```python
from build123d import *

# Parameters (mm, degrees)
ESBO_O1_R                    = 100
ESBO_O1_R_2                  = 27.5
RESSALTO_EXTRUS_O1_DEPTH     = 65
CORTE_EXTRUS_O1_START        = -5
ESBO_O2_R                    = 100
ESBO_O2_R_2                  = 42.5
CORTE_EXTRUS_O1_DEPTH        = 55
CORTE_EXTRUS_O2_DEPTH        = 157.3
FILETE1_R                    = 10
PADR_OCIRCULAR1_COUNT        = 6
FILETE1_OF_PADR_OCIRCULAR1_R = 10
ESBO_O4_R                    = 4
CORTE_EXTRUS_O3_DEPTH        = 157.3
PADR_OCIRCULAR2_COUNT        = 22


with BuildPart() as part:
    # Esboço1 → Ressalto-extrusão1 (new body)
    with BuildSketch(Plane.XY):
        Circle(ESBO_O1_R)
        Circle(ESBO_O1_R_2, mode=Mode.SUBTRACT)
    extrude(amount=RESSALTO_EXTRUS_O1_DEPTH)

    # Esboço2 → Corte-extrusão1 (cut)
    with BuildSketch(Plane.XY.offset(65).offset(CORTE_EXTRUS_O1_START)):
        Circle(ESBO_O2_R)
        Circle(ESBO_O2_R_2, mode=Mode.SUBTRACT)
    extrude(amount=-CORTE_EXTRUS_O1_DEPTH, mode=Mode.SUBTRACT)

    # Esboço3 → Corte-extrusão2 (cut)
    with BuildSketch(Plane.XY.offset(65)):
        with BuildLine():
            ThreePointArc((0, 87.5), (-33.484800332, 80.839459095), (-61.871843354, 61.871843354))
            Line((-61.871843354, 61.871843354), (-32.082845763, 44.673157576))
            ThreePointArc((-32.082845763, 44.673157576), (-21.04758878, 50.813374288), (-8.90269486, 54.274690457))
            Line((-8.90269486, 54.274690457), (0, 87.5))
        make_face()
    corte_extrus_o2 = extrude(amount=-CORTE_EXTRUS_O2_DEPTH, mode=Mode.SUBTRACT)

    # Filete1
    filete1_edges = [part.edges().sort_by_distance(p)[0] for p in [
        (0, 87.5, 2.5),
        (0, 87.5, 62.5),
        (-8.90269486, 54.274690457, 2.5),
        (-8.90269486, 54.274690457, 62.5),
        (-32.082845763, 44.673157576, 2.5),
        (-32.082845763, 44.673157576, 62.5),
        (-61.871843354, 61.871843354, 2.5),
        (-61.871843354, 61.871843354, 62.5),
    ]]
    fillet(filete1_edges, radius=FILETE1_R)

    # PadrãoCircular1: Corte-extrusão2 ×6 about axis
    padr_ocircular1_axis = Axis((0, 0, 0), (0, 0, 1))
    for i in range(1, PADR_OCIRCULAR1_COUNT):
        add(corte_extrus_o2.rotate(padr_ocircular1_axis, i * 360 / PADR_OCIRCULAR1_COUNT), mode=Mode.SUBTRACT)

    # Filete1 of PadrãoCircular1
    filete1_of_padr_ocircular1_edges = [part.edges().sort_by_distance(p)[0] for p in [
        (-75.777222831, 43.75, 2.5),
        (-75.777222831, 43.75, 62.5),
        (-51.454608149, 19.427385317, 2.5),
        (-51.454608149, 19.427385317, 62.5),
        (-54.729512209, -5.447980668, 2.5),
        (-54.729512209, -5.447980668, 62.5),
        (-84.5185098, -22.646666446, 2.5),
        (-84.5185098, -22.646666446, 62.5),
        (-75.777222831, -43.75, 2.5),
        (-75.777222831, -43.75, 62.5),
        (-42.551913288, -34.84730514, 2.5),
        (-42.551913288, -34.84730514, 62.5),
        (-22.646666446, -50.121138244, 2.5),
        (-22.646666446, -50.121138244, 62.5),
        (-22.646666446, -84.5185098, 2.5),
        (-22.646666446, -84.5185098, 62.5),
        (0, -87.5, 2.5),
        (0, -87.5, 62.5),
        (8.90269486, -54.274690457, 2.5),
        (8.90269486, -54.274690457, 62.5),
        (32.082845763, -44.673157576, 2.5),
        (32.082845763, -44.673157576, 62.5),
        (61.871843354, -61.871843354, 2.5),
        (61.871843354, -61.871843354, 62.5),
        (75.777222831, -43.75, 2.5),
        (75.777222831, -43.75, 62.5),
        (51.454608149, -19.427385317, 2.5),
        (51.454608149, -19.427385317, 62.5),
        (54.729512209, 5.447980668, 2.5),
        (54.729512209, 5.447980668, 62.5),
        (84.5185098, 22.646666446, 2.5),
        (84.5185098, 22.646666446, 62.5),
        (75.777222831, 43.75, 2.5),
        (75.777222831, 43.75, 62.5),
        (42.551913288, 34.84730514, 2.5),
        (42.551913288, 34.84730514, 62.5),
        (22.646666446, 50.121138244, 2.5),
        (22.646666446, 50.121138244, 62.5),
        (22.646666446, 84.5185098, 2.5),
        (22.646666446, 84.5185098, 62.5),
    ]]
    fillet(filete1_of_padr_ocircular1_edges, radius=FILETE1_OF_PADR_OCIRCULAR1_R)

    # Esboço4 → Corte-extrusão3 (cut)
    with BuildSketch(Plane.XY.offset(65)):
        with Locations((0, 35)):
            Circle(ESBO_O4_R)
    corte_extrus_o3 = extrude(amount=-CORTE_EXTRUS_O3_DEPTH, mode=Mode.SUBTRACT)

    # PadrãoCircular2: Corte-extrusão3 ×22 about axis
    padr_ocircular2_axis = Axis((0, 0, 0), (0, 0, 1))
    for i in range(1, PADR_OCIRCULAR2_COUNT):
        add(corte_extrus_o3.rotate(padr_ocircular2_axis, i * 360 / PADR_OCIRCULAR2_COUNT), mode=Mode.SUBTRACT)


solid = part.part
```
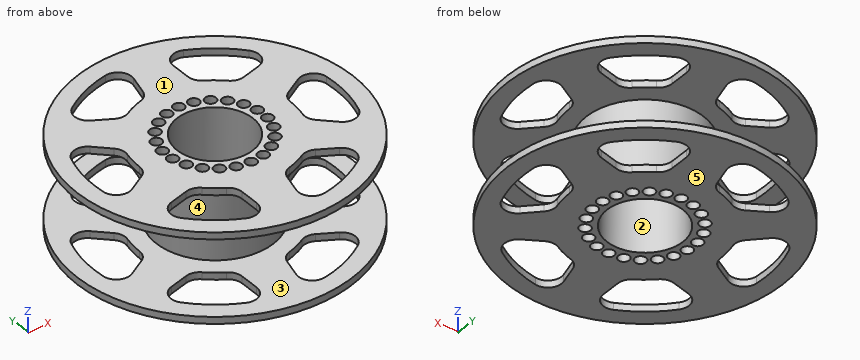
Here's how the part is built. I have some questions about the finished solid (model axes, mm). Face numbers are marked on the shaded views. A direction names the side the tool comes from. Round coordinates to 2 decimals unless told otherwise and drop trailing zeros. Order: outer loops, then holes, each group sorted by start corner. A loop starts at its lowest first (then second) coordinate and runs counter-clockwise, first axis right, second up. Notation, with made-up numbers: M 6,-15 L 61,-15 A23 cw 61,19 Z; hole C -6.75,8.5 d11. An arc over 180 degrees is marked long. Answer in a Markdown table with one row per item.
Item 1: If I drill on L1, parallel to Z at x = -27.5, y = 42.5; L2, parallel to Y at x = 35, z = 38.5; L3, parallel to Y at x = 21.5, z = 56.5, over which ranges is the centre line in solid material (lowest first)? Write a range as from..to.
A:
| item | result |
|---|---|
| L1 | z = 0..5, 60..65 |
| L2 | y = -24.11..-16.99, -12.09..-8.97, -1..1, 8.97..12.09, 16.99..24.11 |
| L3 | y = -36.66..-32.5, -26.39..-17.15, 17.15..26.39, 32.5..36.66 |
Item 2: Imagine slicing it at B-B, the plane y = 77. Write out the boundary of the cut face in (x, z).
A:
| item | result |
|---|---|
| outline | M -63.8,0 L -41.56,0 L -41.56,5 L -63.8,5 Z; M -63.8,60 L -41.56,60 L -41.56,65 L -63.8,65 Z; M -3.36,0 L 25.23,0 L 25.23,5 L -3.36,5 Z; M -3.36,60 L 25.23,60 L 25.23,65 L -3.36,65 Z; M 41.56,0 L 63.8,0 L 63.8,5 L 41.56,5 Z; M 41.56,60 L 63.8,60 L 63.8,65 L 41.56,65 Z |
Item 3: For the marked faces 4 and 5, which set-ups out of +Z, -Z, +X, -X, +Y, -Y let a thin tool reach every point of the face, with its end or its side?
A:
| item | result |
|---|---|
| face 4 | none |
| face 5 | -Z, +X, -X, +Y, -Y |
Item 4: Imagine slicing it at C-C, the plane z = 54.5. State how many separate pieces and enclosed holes the cut face has, and give its area (3 significant figures).
A:
| item | result |
|---|---|
| separate pieces | 1 |
| enclosed holes | 23 |
| area | 2,190 mm2 |
Item 5: I'm going to push flat-ended pins straight in: pin 1 (6.5 mm diameter, centred on x = 9.86, y = -33.58, fed in from +Z); pin 2 (1.5 mm diameter, centred on y = -61, z = 2.5, fed in from -X); pin 3 (4 mm diameter, centred on y = -64, z = 61.5, fed in from -X); pin 4 (8 mm diameter, centred on y = -23, z = 57, fed in from -X). Where does each tip first touch, or does it pass through?
A:
| item | result |
|---|---|
| pin 1 | passes through |
| pin 2 | stops at x = -79.81 |
| pin 3 | stops at x = -78.46 |
| pin 4 | stops at x = -97.91 |
Item 6: Thinking about a two-plate mould opening in Z: for the marked faces 1, 2 and 3, which applies, +Z half, -Z half, draft (parallel to the pull), parting line (faces both ways), or undercut?
A:
| item | result |
|---|---|
| face 1 | +Z half |
| face 2 | draft |
| face 3 | undercut |
Item 7: Imagine slicing it at A-A, the plane x = 0. Write out the boundary of the cut face in (y, z).
A:
| item | result |
|---|---|
| outline | M -100,0 L -39,0 L -39,65 L -100,65 L -100,60 L -42.5,60 L -42.5,5 L -100,5 Z; M -31,0 L -27.5,0 L -27.5,65 L -31,65 Z; M 27.5,0 L 31,0 L 31,65 L 27.5,65 Z; M 39,0 L 100,0 L 100,5 L 42.5,5 L 42.5,60 L 100,60 L 100,65 L 39,65 Z |
